from build123d import *

# Parameters (mm, degrees)
CROQUIS1_W              = 8
CROQUIS1_H              = 13
SALIENTE_EXTRUIR1_DEPTH = 15
CROQUIS3_R              = 11
CORTAR_EXTRUIR1_DEPTH   = 15
CROQUIS4_R              = 2.5
CORTAR_EXTRUIR2_DEPTH   = 30
REDONDEO1_R             = 10
CROQUIS5_R              = 2.5
CORTAR_EXTRUIR3_DEPTH   = 2
SKETCH2_R               = 11
SKETCH2_R_2             = 4
BOSS_EXTRUDE1_DEPTH     = 3
SKETCH3_R               = 11
SKETCH3_R_2             = 4
BOSS_EXTRUDE2_DEPTH     = 3
SKETCH4_W               = 3.5
SKETCH4_H               = 2
SKETCH4_W_2             = 4
CUT_EXTRUDE1_DEPTH      = 31
SKETCH5_W               = 30
SKETCH5_H               = 19
CUT_EXTRUDE2_DEPTH      = 0.7


with BuildPart() as part:
    # Croquis1 → Saliente-Extruir1 (new body, symmetric)
    with BuildSketch(Plane.XY):
        Polygon((-15, -2), (-7, -2), (-7, -15), (-15, -15), (-15, -17), (-8, -17), (-8, -33), (-6, -33), (-6, -17), (6, -17), (6, -33), (8, -33), (8, -17), (15, -17), (15, -15), (7, -15), (7, -2), (15, -2), (15, 2), (7, 2), (7, 15), (15, 15), (15, 17), (-15, 17), (-15, 15), (-7, 15), (-7, 2), (-15, 2), align=None)
        with Locations((0, 8.5)):
            Rectangle(CROQUIS1_W, CROQUIS1_H, mode=Mode.SUBTRACT)
        with Locations((0, -8.5)):
            Rectangle(CROQUIS1_W, CROQUIS1_H, mode=Mode.SUBTRACT)
    extrude(amount=SALIENTE_EXTRUIR1_DEPTH, both=True)

    # Croquis3 → Cortar-Extruir1 (cut, symmetric)
    with BuildSketch(Plane(origin=(0, 0, 0), x_dir=(0, 0, -1), z_dir=(1, 0, 0))):
        Circle(CROQUIS3_R)
    extrude(amount=CORTAR_EXTRUIR1_DEPTH, both=True, mode=Mode.SUBTRACT)

    # Croquis4 → Cortar-Extruir2 (cut)
    with BuildSketch(Plane(origin=(8, 0, 0), x_dir=(0, 0, -1), z_dir=(1, 0, 0))):
        with Locations((-8, -25)):
            Circle(CROQUIS4_R)
        with Locations((8, -25)):
            Circle(CROQUIS4_R)
    extrude(amount=-CORTAR_EXTRUIR2_DEPTH, mode=Mode.SUBTRACT)

    # Redondeo1
    redondeo1_edges = [part.edges().sort_by_distance(p)[0] for p in [
        (7, -33, -15),
        (-7, -33, -15),
        (-7, -33, 15),
        (7, -33, 15),
    ]]
    fillet(redondeo1_edges, radius=REDONDEO1_R)

    # Croquis5 → Cortar-Extruir3 (cut)
    with BuildSketch(Plane(origin=(0, 17, 0), x_dir=(1, 0, 0), z_dir=(0, 1, 0))):
        with Locations((-11, 0)):
            Circle(CROQUIS5_R)
        with Locations((11, 0)):
            Circle(CROQUIS5_R)
    extrude(amount=-CORTAR_EXTRUIR3_DEPTH, mode=Mode.SUBTRACT)

    # Sketch2 → Boss-Extrude1 (add)
    with BuildSketch(Plane(origin=(7, 0, 0), x_dir=(0, 0, -1), z_dir=(1, 0, 0))):
        Circle(SKETCH2_R)
        Circle(SKETCH2_R_2, mode=Mode.SUBTRACT)
    extrude(amount=-BOSS_EXTRUDE1_DEPTH)

    # Sketch3 → Boss-Extrude2 (add)
    with BuildSketch(Plane.ZY.offset(7)):
        Circle(SKETCH3_R)
        Circle(SKETCH3_R_2, mode=Mode.SUBTRACT)
    extrude(amount=-BOSS_EXTRUDE2_DEPTH)

    # Sketch4 → Cut-Extrude1 (cut, through all)
    with BuildSketch(Plane(origin=(0, 0, -15), x_dir=(-1, 0, 0), z_dir=(0, 0, -1))):
        with Locations((-13.25, -16)):
            Rectangle(SKETCH4_W, SKETCH4_H)
        with Locations((13, -16)):
            Rectangle(SKETCH4_W_2, SKETCH4_H)
    extrude(amount=-CUT_EXTRUDE1_DEPTH, mode=Mode.SUBTRACT)

    # Sketch5 → Cut-Extrude2 (cut)
    with BuildSketch(Plane.ZY.offset(15)):
        with Locations((0, 7.5)):
            Rectangle(SKETCH5_W, SKETCH5_H)
    extrude(amount=-CUT_EXTRUDE2_DEPTH, mode=Mode.SUBTRACT)


solid = part.part
For this review, take the finished solid that the model builds, in its own axes (mm). A direction names the side the tool comes from. Round coordinates to 2 decimals unless told otherwise and drop trailing zeros. Write each loop counter-clockwise with the first axis right and the second up, starting at its lowest first coordinate (ties: lowest second). Pieces come first, ordered by that corner, then holes. Notation, with made-up numbers: (-28.75, 78) -> (18.25, 78) arc R21 cw to (18.25, 86) -> close; hole circle Ø9 at (64, 86). An arc over 180 degrees is marked (long way). Use CSV: the item, a comma, the result in double quotes.
(1) Consider section D-D, the plane x = 10.5. Give the boundary of the cut face in (y, z).
Computed values:
outline,"(-17, -15) -> (-15, -15) -> (-15, 15) -> (-17, 15) -> close; (-2, -15) -> (2, -15) -> (2, -10.82) arc R11 cw to (-2, -10.82) -> close; (-2, 10.82) arc R11 cw to (2, 10.82) -> (2, 15) -> (-2, 15) -> close; (15, -15) -> (17, -15) -> (17, -2.45) -> (15, -2.45) -> close; (15, 2.45) -> (17, 2.45) -> (17, 15) -> (15, 15) -> close"
(2) Consider section C-C, the plane x = 1. Give the boundary of the cut face in (y, z).
Computed values:
outline,"(-17, -15) -> (-15, -15) -> (-15, 15) -> (-17, 15) -> close; (-2, -15) -> (2, -15) -> (2, -10.82) arc R11 cw to (-2, -10.82) -> close; (-2, 10.82) arc R11 cw to (2, 10.82) -> (2, 15) -> (-2, 15) -> close; (15, -15) -> (17, -15) -> (17, 15) -> (15, 15) -> close"
(3) To check wall thickness, follow L1, parallel to X at y = 13.5, z = 9.5; L2, parallel to X at y = -19, z = 1; L3, parallel to Y at x = -7.3, z = -8. State the ranges of each line that lie inside material, in increasing order. Write a range as [from, to].
Computed values:
L1,"[-7, -4], [4, 7]"
L2,"[-8, -6], [6, 8]"
L3,"[-32.54, -27.5], [-22.5, -15], [15, 17]"
(4) For faces 1 (the face through (-11, 2, -13)), 2 (the face through (11, -2, -13)), 3 (the face through (0, 0, 11)), 4 (the face through (-6, -25, 0)), list the 3-axis set-ups (+Z, -Z, +X, -X, +Y, -Y) from which the entire face can be reached by the end or side of a thin tool; tool diameter is ignored.
Computed values:
face 1,"+Z, -Z, -X"
face 2,"+Z, -Z, +X"
face 3,"none"
face 4,"+Z, -Z, -Y"
(5) Consider section B-B, the plane z = -8. Give the number of separate pieces and of enclosed holes in the cut face, plus the area to 3 significant figures.
Computed values:
separate pieces,"3"
enclosed holes,"1"
area,"326 mm²"
(6) Draft analysis for pull direction X (two halves, no side actions). For faces 5 (the face through (-11, -16, 0)), 6 (the face through (0, 15, 0)), 7 (the face through (-11, 0, -11)), state which applies: +X half, -X half, draft (parallel to the pull), parting line (faces both ways), or undercut.
Computed values:
face 5,"-X half"
face 6,"undercut"
face 7,"draft"
(7) Clearance check with flat-ended pins moving along their axes: P1, Ø10, axis at x = -1.5, y = -9, coming from the -Z side; P2, Ø6, axis at x = -1, z = -4.5, coming from the -Y side; P3, Ø15, axis at y = -4.5, z = 0, coming from the -X side; P4, Ø6, axis at y = -25, z = 8, coming from the -X side. State where each tip first meets the part, or that it passes through.
Computed values:
P1,"z = -15"
P2,"y = -17"
P3,"x = -7"
P4,"x = -8"
(8) Consider section A-A, the plane y = 0. Give the boundary of the cut face in (x, z), plus the area to 3 significant figures.
Computed values:
outline,"(-14.3, -15) -> (15, -15) -> (15, -11) -> (7, -11) -> (7, -4) -> (4, -4) -> (4, -11) -> (-4, -11) -> (-4, -4) -> (-7, -4) -> (-7, -11) -> (-14.3, -11) -> close; (-14.3, 11) -> (-7, 11) -> (-7, 4) -> (-4, 4) -> (-4, 11) -> (4, 11) -> (4, 4) -> (7, 4) -> (7, 11) -> (15, 11) -> (15, 15) -> (-14.3, 15) -> close"
area,"318 mm²"
